```python
from build123d import *

# Parameters (mm, degrees)
SKETCH1_W           = 50
SKETCH1_H           = 70
BOSS_EXTRUDE1_DEPTH = 40
SKETCH2_W           = 50
SKETCH2_H           = 10
CUT_EXTRUDE1_DEPTH  = 20


with BuildPart() as part:
    # Sketch1 → Boss-Extrude1 (new body)
    with BuildSketch(Plane.XY):
        Rectangle(SKETCH1_W, SKETCH1_H)
    extrude(amount=-BOSS_EXTRUDE1_DEPTH)

    # Sketch2 → Cut-Extrude1 (cut)
    with BuildSketch(Plane.XY):
        with Locations((0, 20)):
            Rectangle(SKETCH2_W, SKETCH2_H)
    extrude(amount=-CUT_EXTRUDE1_DEPTH, mode=Mode.SUBTRACT)


solid = part.part
```
Part model, mm, in its own coordinate system. A direction names the side the tool comes from. Give positions to 0.01 mm unless a question says otherwise; leave off trailing zeros. Loops run counter-clockwise (first coordinate to the right, second up) from the corner with the lowest first, then second, coordinate; pieces in that order, holes last. Notation, with made-up numbers: M 82.5,61 L 139.5,61 A23 cw 139.5,76 Z; hole C -33,-9 d11. An arc over 180 degrees is marked long. Return JSON: item names as keys, results as strings.
1) Pull direction Y, two halves, no side cores. Call faces 1 (the face through (0, 35, -20)), 2 (the face through (0, 0, -40)), 3 (the face through (0, 20, -20)): released by +Y, released by -Y, zero draft, split by the parting line, or undercut.
Calculated:
{"face 1": "released by +Y", "face 2": "zero draft", "face 3": "undercut"}
2) Saw through at A-A, the plane z = -13. List the corners of the cut face in (x, y).
Calculated:
{"outline": "M -25,-35 L 25,-35 L 25,15 L -25,15 Z; M -25,25 L 25,25 L 25,35 L -25,35 Z"}
3) Flat gauge pin, fed straight in: pin 1 Ø10 at (x, y) = (17, -10) entering from +Z. Where does the tip first touch, or does it go through?
Calculated:
{"pin 1": "stops at z = 0"}
4) Saw through at B-B, the plane x = 5.5. List the corners of the cut face in (y, z), then the cut area to 3 significant figures.
Calculated:
{"outline": "M -35,-40 L 35,-40 L 35,0 L 25,0 L 25,-20 L 15,-20 L 15,0 L -35,0 Z", "area": "2,600 mm2"}
5) Drill centre lines: line 1 (Y direction, x = -19, z = -8); line 2 (Z direction, x = -22, y = 18.5). Where is each one in solid material? Low to high.
Calculated:
{"line 1": "y = -35 to 15, 25 to 35", "line 2": "z = -40 to -20"}
6) 3-axis set-ups, long thin cutter, end or side, ignore diameter. For faces 4 (the face through (0, -10, 0)), 5 (the face through (0, 15, -10)): which of +Z, -Z, +X, -X, +Y, -Y reach the whole face in a straight line?
Calculated:
{"face 4": "+Z, +X, -X, +Y, -Y", "face 5": "+Z, +X, -X"}
